Job drawing, mm, ordinate dimensions from the low corner. One solid piece. Round coordinates to 2 decimals unless told otherwise and drop trailing zeros. Order: outer loops, then holes, each group sorted by start corner. A loop starts at its lowest first (then second) coordinate and runs counter-clockwise, first axis right, second up. Notation, with made-up numbers: (-16.75, 65) - (19.25, 65) arc R22 cw to (19.25, 88) - close; hole circle Ø2 at (1.5, 78.5). An arc over 180 degrees is marked (long way). Write each question's results on one line, items separated by ' | '. Start each with the question number.
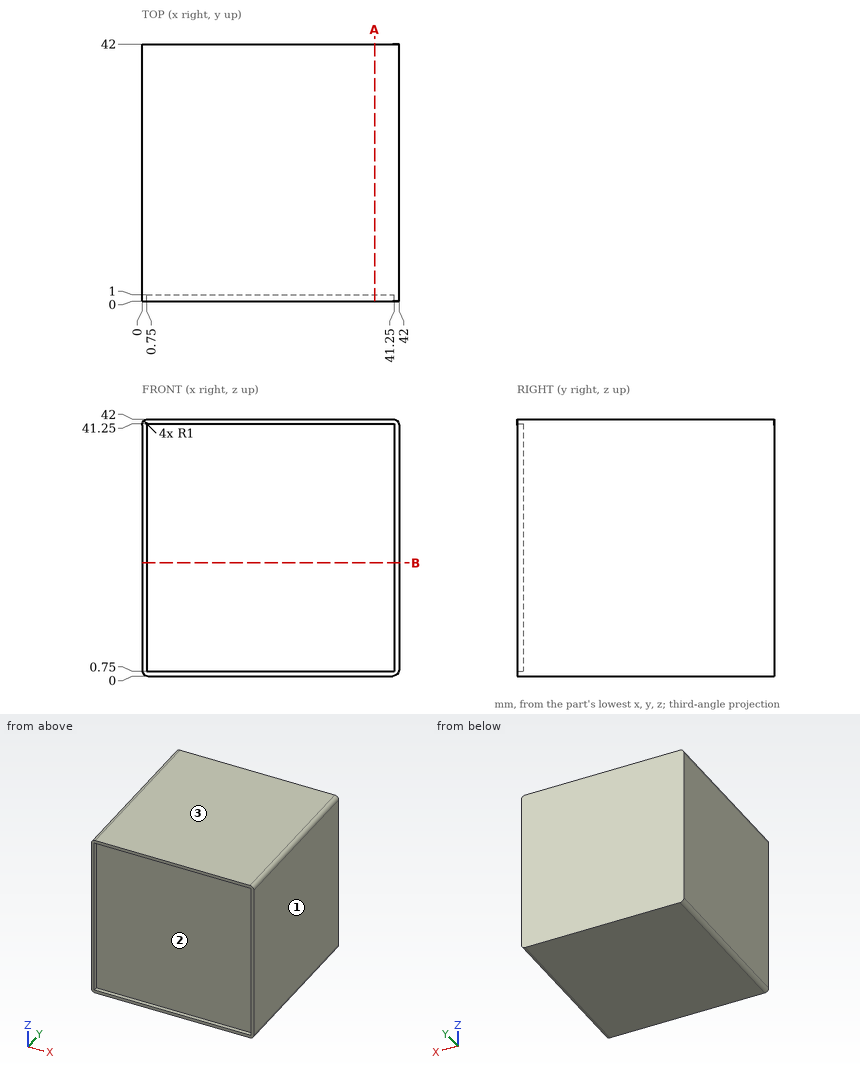
1. Mould opens along X. For the marked faces 1, 2 and 3 say: pulls with the +X half, pulls with the -X half, needs draft (parallel to the pull), parting line crosses it, or undercut.
2. Wall check: line 1 (Y direction, x = 21, z = 36). Give the ranges that are in metal, low to high. Write a range as from..to.
3. Cut at A-A (x = 38). List the corners of the cut face in (y, z).
4. Flat gauge pin, fed straight in: pin 1 Ø6 at (x, z) = (9.5, 17) entering from -Y. Where does the tip first touch, or does it go through?
5. Cut at B-B (z = 18.5). List the corners of the cut face in (x, y).
A:
1) face 1: pulls with the +X half | face 2: undercut | face 3: needs draft
2) line 1: y = 1..42
3) outline: (0, 0) - (42, 0) - (42, 42) - (0, 42) - (0, 41.25) - (1, 41.25) - (1, 0.75) - (0, 0.75) - close
4) pin 1: stops at y = 1
5) outline: (0, 0) - (0.75, 0) - (0.75, 1) - (41.25, 1) - (41.25, 0) - (42, 0) - (42, 42) - (0, 42) - close
